from build123d import *

# Parameters (mm, degrees)
F1_DEPTH = 1.5
F3_DEPTH = 1.5
F5_DEPTH = 1.5


with BuildPart() as f1:
    # F0 (on Top) → F1 (new body)
    with BuildSketch(Plane.XY):
        with BuildLine():
            Line((-38.65, -29), (38.65, -29))
            ThreePointArc((38.65, -29), (43.140128, -27.140128), (45, -22.65))
            Line((45, -22.65), (45, 22.65))
            ThreePointArc((45, 22.65), (43.140128, 27.140128), (38.65, 29))
            Line((38.65, 29), (-38.65, 29))
            ThreePointArc((-38.65, 29), (-43.140128, 27.140128), (-45, 22.65))
            Line((-45, 22.65), (-45, -22.65))
            ThreePointArc((-45, -22.65), (-43.140128, -27.140128), (-38.65, -29))
        make_face()
    extrude(amount=F1_DEPTH)

    # F2 (on face) → F3 (join)
    with BuildSketch(Plane.XY.offset(1.5)):
        with BuildLine():
            ThreePointArc((38.65, -29), (43.140128, -27.140128), (45, -22.65))
            Line((45, -22.65), (45, 12.129959))
            Line((45, 12.129959), (-45, 12.129959))
            Line((-45, 12.129959), (-45, -22.65))
            ThreePointArc((-45, -22.65), (-43.140128, -27.140128), (-38.65, -29))
            Line((-38.65, -29), (38.65, -29))
        make_face()
    extrude(amount=F3_DEPTH)

    # F4 (on face) → F5 (join)
    with BuildSketch(Plane(origin=(0, 0, 0), x_dir=(1, 0, 0), z_dir=(0, 0, -1))):
        with BuildLine():
            ThreePointArc((-45, -12.129959), (-0.068582, -0.00037), (45, -11.609941))
            Line((45, -11.609941), (45, 22.65))
            ThreePointArc((45, 22.65), (43.140128, 27.140128), (38.65, 29))
            Line((38.65, 29), (-38.65, 29))
            ThreePointArc((-38.65, 29), (-43.140128, 27.140128), (-45, 22.65))
            Line((-45, 22.65), (-45, -12.129959))
        make_face()
    extrude(amount=F5_DEPTH)


solid = f1.part
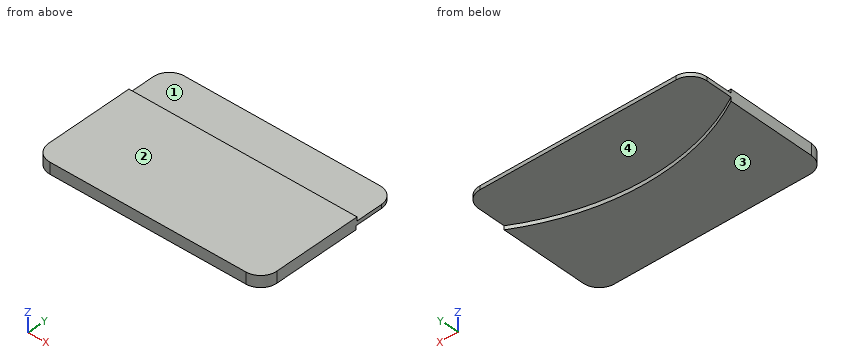
The model under review builds one solid part; all positions refer to its coordinate system, in mm. Face numbers are marked on the shaded views. A direction names the side the tool comes from. Round coordinates to 2 decimals unless told otherwise and drop trailing zeros. Write each loop counter-clockwise with the first axis right and the second up, starting at its lowest first coordinate (ties: lowest second). Pieces come first, ordered by that corner, then holes. Notation, with made-up numbers: M 1,-31 L 55,-31 A22 cw 55,-3 Z; hole C 15,46.25 d7. An arc over 180 degrees is marked long. Use a Markdown table: item, result. Add a question column.
Q1. Insertion check: pin 1 (23 mm diameter, centred on x = -9.5, y = 19, fed in from -Z). The pin has a flat end and moves straight along its axis. Give the tip position at first contact, or say it passes through.
Q2. Machinability: for the marked faces 1 and 2, which of the approach directions +Z, -Z, +X, -X, +Y, -Y give a long, thin tool a straight path to every point of the face, cutting with its end or side? Answer none if there is none.
Q3. We need section B-B, the plane y = 16. State the section outline as (x, z) points, plus the area to 3 significant figures.
Q4. To check wall thickness, follow line 1 (Z direction, x = 0.5, y = 22.5); line 2 (Y direction, x = -4, z = 2.2); line 3 (Y direction, x = 30.5, z = -0.6). State the ranges of each line that lie inside material, in increasing order.
Q5. We need section C-C, the plane x = -1.5. State the section outline as (y, z) points.
Q6. The part is to be moulded in two halves that separate along X. For the marked faces 3 and 4, say which applies: pulls with the +X half, pulls with the -X half, needs draft (parallel to the pull), parting line crosses it, or undercut.
Q7. We need section A-A, the plane x = 10.5. State the section outline as (y, z) points, plus the area to 3 significant figures.
Findings below:
| question | item | result |
|---|---|---|
| 1 | pin 1 | stops at z = 0 |
| 2 | face 1 | +Z, +X, -X, +Y |
| 2 | face 2 | +Z, +X, -X, +Y, -Y |
| 3 | outline | M -45,0 L 45,0 L 45,1.5 L -45,1.5 Z |
| 3 | area | 135 mm² |
| 4 | line 1 | z = 0 to 1.5 |
| 4 | line 2 | y = -29 to 12.13 |
| 4 | line 3 | y = -29 to 5.09 |
| 5 | outline | M -29,-1.5 L 0.02,-1.5 L 0.02,0 L 29,0 L 29,1.5 L 12.13,1.5 L 12.13,3 L -29,3 Z |
| 6 | face 3 | needs draft |
| 6 | face 4 | undercut |
| 7 | outline | M -29,-1.5 L 0.55,-1.5 L 0.55,0 L 29,0 L 29,1.5 L 12.13,1.5 L 12.13,3 L -29,3 Z |
| 7 | area | 193 mm² |
